Geometry check sheet. Reference: the model listing, model coordinates, mm. Give positions to 0.01 mm unless a question says otherwise; leave off trailing zeros. Order: outer loops, then holes, each group sorted by start corner. A loop starts at its lowest first (then second) coordinate and runs counter-clockwise, first axis right, second up.
Autodesk Inventor part; units mm, degrees
ref_plane "YZ Plane" through (0, 0, 0) normal (1, 0, 0) x (0, 1, 0)
ref_plane "XZ Plane" through (0, 0, 0) normal (0, 1, 0) x (-1, 0, 0)
ref_plane "XY Plane" through (0, 0, 0) normal (0, 0, 1) x (1, 0, 0)
sketch "Sketch1" plane through (0, 0, 0) normal (0, 0, 1) x (1, 0, 0)
  line L0 (17.5196, 21.1512) -> (-17.5142, 21.1512)
  line L1 (-21.1533, 17.5121) -> (-21.1533, -17.5122)
  line L2 (-17.5142, -21.1513) -> (17.5196, -21.1513)
  line L3 (21.1587, -17.5122) -> (21.1587, 17.5121)
  line L4 (21.1533, 21.1533) -> (-21.1467, -21.1467) construction
  line L5 (-21.1598, 21.1533) -> (21.1533, -21.1467) construction
  line L6 (-17.691, 21.078) -> (-21.08, 17.6889)
  line L7 (17.6964, 21.078) -> (21.0855, 17.6889)
  line L8 (21.0855, -17.689) -> (17.6964, -21.0781)
  line L9 (-17.691, -21.0781) -> (-21.08, -17.689)
  arc A0 (-17.5142, 21.1512) -> (-17.691, 21.078) centre (-17.5142, 20.9012) ccw
  arc A1 (-21.08, 17.6889) -> (-21.1533, 17.5121) centre (-20.9033, 17.5121) ccw
  arc A2 (17.6964, 21.078) -> (17.5196, 21.1512) centre (17.5196, 20.9012) ccw
  arc A3 (21.1587, 17.5121) -> (21.0855, 17.6889) centre (20.9087, 17.5121) ccw
  arc A4 (21.0855, -17.689) -> (21.1587, -17.5122) centre (20.9087, -17.5122) ccw
  arc A5 (17.5196, -21.1513) -> (17.6964, -21.0781) centre (17.5196, -20.9013) ccw
  arc A6 (-17.691, -21.0781) -> (-17.5142, -21.1513) centre (-17.5142, -20.9013) ccw
  arc A7 (-21.1533, -17.5122) -> (-21.08, -17.689) centre (-20.9033, -17.5122) ccw
  point P0 (0, 0)
  point P1 (-17.6177, 21.1512)
  point P2 (-21.1533, 17.6156)
  dimension "d0" = 42.3
  dimension "d1" = 42.3
  dimension "d2" = 5
  dimension "d3" = 45
  dimension "d4" = 0.25
extrude "Extrusion1" add sketch "Sketch1" along normal blind 40
sketch "Sketch2" plane through (0, 0, 40) normal (0, 0, 1) x (1, 0, 0)
  circle A0 centre (0, 0) radius 11
  circle A1 centre (0, 0) radius 5
  dimension "d7" = 22
  dimension "d8" = 10
extrude "Extrusion2" add sketch "Sketch2" along normal blind 2
sketch "Sketch3" plane through (0, 0, 40) normal (0, 0, 1) x (1, 0, 0)
  circle A0 centre (0, 0) radius 11
  line L0 (-15.5, -15.5) -> (15.5, -15.5) construction
  line L1 (15.5, -15.5) -> (15.5, 15.5) construction
  line L2 (15.5, 15.5) -> (-15.5, 15.5) construction
  line L3 (-15.5, 15.5) -> (-15.5, -15.5) construction
  line L4 (-15.5, -15.5) -> (15.5, 15.5) construction
  line L5 (15.5, -15.5) -> (-15.5, 15.5) construction
  dimension "d11" = 31
  dimension "d12" = 31
hole "Hole1" at (-15.5, 15.5, 40) at (15.5, 15.5, 40) at (15.5, -15.5, 40) at (-15.5, -15.5, 40) direction (0, 0, -1) diameter 2.459 depth 4.5 tip angle 118
sketch "Sketch4" plane through (0, 0, 40) normal (0, 0, 1) x (1, 0, 0)
  circle A0 centre (0, 0) radius 5
  circle A1 centre (0, 0) radius 4
  dimension "d20" = 8
extrude "Extrusion3" add sketch "Sketch4" along normal blind 350 contours A1
properties part number "motor"
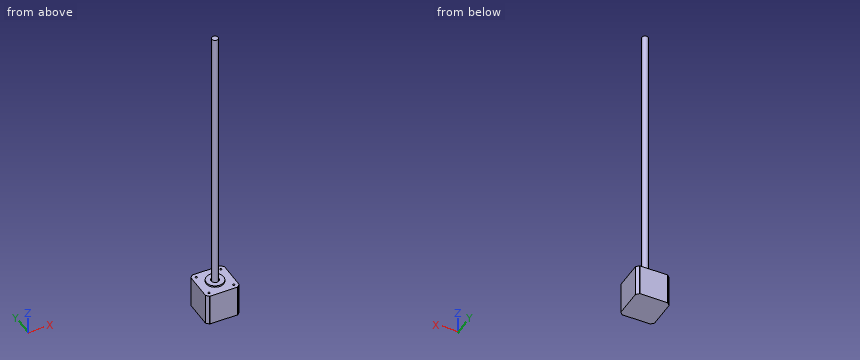
Q1. Gauge pin test, flat ends, axial feed: P1, Ø8, axis at x = 10.5, z = 237.5, coming from the -Y side; P2, Ø5, axis at x = -12.5, y = 16, coming from the +Z side; P3, Ø2, axis at y = 1, z = 259.5, coming from the -X side; P4, Ø2, axis at x = -15.5, y = -15.5, coming from the +Z side. Record the tip position at first contact, or that the pin passes through.
Q2. Thickness scan on L1, parallel to Y at x = -15.5, z = 38.8; L2, parallel to Y at x = 0, z = 41; L3, parallel to X at y = 15.5, z = 38.6. Record the ranges inside material, lowest first.
Q3. Cross-section at A-A, the plane y = 0. Record the boundary of the cut face in (x, z), and give its area (3 significant figures).
Q4. Cross-section at B-B, the plane z = 55. Record the boundary of the cut face in (x, y).
Answers follow:
1. P1: passes through
1. P2: stops at z = 40
1. P3: stops at x = -4
1. P4: stops at z = 35.36
2. L1: y = -21.15 to -16.73, -14.27 to 14.27, 16.73 to 21.15
2. L2: y = -11 to -5, -4 to 4, 5 to 11
2. L3: x = -21.15 to -16.73, -14.27 to 14.27, 16.73 to 21.16
3. outline: (-21.15, 0) - (21.16, 0) - (21.16, 40) - (11, 40) - (11, 42) - (5, 42) - (5, 40) - (4, 40) - (4, 390) - (-4, 390) - (-4, 40) - (-5, 40) - (-5, 42) - (-11, 42) - (-11, 40) - (-21.15, 40) - close
3. area: 4,520 mm2
4. outline: circle Ø8 at (0, 0)
